Verification items for the finished model (mm, model axes). A direction names the side the tool comes from. Give positions to 0.01 mm unless a question says otherwise; leave off trailing zeros. Order: outer loops, then holes, each group sorted by start corner. A loop starts at its lowest first (then second) coordinate and runs counter-clockwise, first axis right, second up. Notation, with made-up numbers: (-25, 53) -> (33, 53) arc R4 ccw to (33, 58) -> close; hole circle Ø1 at (46.25, 65.5). An arc over 180 degrees is marked (long way). Return JSON: item names as keys, results as strings. Group by question number.
(1) Tool access check on faces 1 (the face through (-0.356, 0.174, 26.758)), 2 (the face through (0, 1.27, 12)), 3 (the face through (0, 0, 30.48)). Record the directions out of +Z, -Z, +X, -X, +Y, -Y that give a thin tool (end or side, any length) a straight path to the whole face; none if there is none.
(2) Thickness scan on line 1 along Z through (x, y) = (1.25, -0.25); line 2 along Y through (x, z) = (0.25, 11); line 3 along Z through (x, y) = (-0.5, 1). Record the ranges inside material, lowest first.
(3) Release check for a two-part mould opening along Z. For faces 4 (the face through (0, 0, -30.48)), 5 (the face through (0, -0.953, 25)), 6 (the face through (0.039, 1.567, -5.941)) record: pulls with the +Z half, pulls with the -Z half, needs draft (parallel to the pull), parting line crosses it, or undercut.
(4) Depth check by flat-ended pin: pin 1 Ø2.5 at (x, z) = (0, 25.15) entering from +Y; pin 2 Ø3 at (y, z) = (-2, -5.5) entering from -X. Enter the tip coordinate at first touch or a pass-through.
(5) Cross-section at A-A on z = 11. Enter the section's corners in (x, y) (3 decimals).
(6) Cross-section at B-B on z = -8.5. Enter the section's corners in (x, y) (3 decimals).
from build123d import *

# Parameters (mm, degrees)
SKETCH1_R          = 3.175
EXTRUDE1_DEPTH     = 30.48
CHAMFER1_SIZE      = 0.635
EXTRUDE7_DEPTH     = 38.084
FILLET1_R          = 1.5875
FILLET3_R          = 0.79375
FILLET4_R          = 0.1984375
SKETCH14_R         = 1.651
CUT_EXTRUDE1_DEPTH = 2.2225


with BuildPart() as part:
    # Sketch1 → Extrude1 (new body, symmetric)
    with BuildSketch(Plane.XY):
        Circle(SKETCH1_R)
    extrude(amount=EXTRUDE1_DEPTH, both=True)

    # Chamfer1
    chamfer1_edges = [part.edges().sort_by_distance(p)[0] for p in [
        (-3.175, 0, -30.48),
        (-3.175, 0, 30.48),
    ]]
    chamfer(chamfer1_edges, length=CHAMFER1_SIZE)

    # Sketch13 → Extrude7 (cut, through all)
    with BuildSketch(Plane.XY.offset(-6.604)):
        with BuildLine():
            Line((-2.909935566, 1.27), (2.909935566, 1.27))
            ThreePointArc((2.909935566, 1.27), (0, 3.175), (-2.909935566, 1.27))
        make_face()
    extrude(amount=EXTRUDE7_DEPTH, mode=Mode.SUBTRACT)

    # Fillet1
    fillet1_edges = [part.edges().sort_by_distance(p)[0] for p in [
        (0, 1.27, -6.604),
    ]]
    fillet(fillet1_edges, radius=FILLET1_R)

    # Fillet3
    fillet3_edges = [part.edges().sort_by_distance(p)[0] for p in [
        (0, -2.54, 30.48),
        (-0.648683119, -3.108027544, 29.845),
    ]]
    fillet(fillet3_edges, radius=FILLET3_R)

    # Fillet4
    fillet4_edges = [part.edges().sort_by_distance(p)[0] for p in [
        (0, 3.175, -6.604),
        (2.5327835, 1.914584225, -6.29363198),
        (-2.5327835, 1.914584225, -6.29363198),
        (0, 1.27, 30.48),
        (2.909935566, 1.27, 12.249858992),
        (-2.909935566, 1.27, 12.249858992),
        (-2.559573738, 1.27, 30.162672977),
        (2.559573738, 1.27, 30.162672977),
        (2.842060138, 1.27, 29.823974262),
        (-2.842060075, 1.27, 29.823974247),
        (-2.158993926, 1.27, 30.423700487),
        (2.158993926, 1.27, 30.423700487),
    ]]
    fillet(fillet4_edges, radius=FILLET4_R)

    # Sketch14 → Cut-Extrude1 (cut)
    with BuildSketch(Plane(origin=(0, 1.27, 0), x_dir=(1, 0, 0), z_dir=(0, 1, 0))):
        with Locations((0.001765627, -25.146)):
            Circle(SKETCH14_R)
    extrude(amount=-CUT_EXTRUDE1_DEPTH, mode=Mode.SUBTRACT)


solid = part.part
Verdict:
{
 "1": {"face 1": "+Y", "face 2": "+Z, +X, -X, +Y", "face 3": "+Z, +X, -X, +Y, -Y"},
 "2": {"line 1": "-30.48 to 24.07, 26.23 to 30.48", "line 2": "-3.17 to 1.27", "line 3": "-30.48 to 23.57, 26.72 to 30.48"},
 "3": {"face 4": "pulls with the -Z half", "face 5": "undercut", "face 6": "pulls with the +Z half"},
 "4": {"pin 1": "y = -0.95", "pin 2": "x = -3.14"},
 "5": {"outline": "(-2.962, 1.143) arc R3.175 ccw (long way) to (2.962, 1.143) arc R0.198 ccw to (2.777, 1.27) -> (-2.777, 1.27) arc R0.198 ccw to start"},
 "6": {"outline": "circle Ø6.35 at (0, 0)"}
}
